Read the model definition and answer for the solid it produces. Units are mm, in the model's axes. A direction names the side the tool comes from. Coordinates: 2 decimals unless noted, no trailing zeros. Write each loop counter-clockwise with the first axis right and the second up, starting at its lowest first coordinate (ties: lowest second). Pieces come first, ordered by that corner, then holes. Notation, with made-up numbers: (52, -13.5) - (91, -13.5) arc R20 ccw to (91, 6.5) - close; hole circle Ø2 at (63, 86). An arc over 180 degrees is marked (long way). Return JSON: item names as keys, results as strings.
```python
from build123d import *

# Parameters (mm, degrees)
EXTRUSION007_DEPTH = 57.9662962441
EXTRUSION006_DEPTH = 1


with BuildPart() as extrusion007:
    # Wire001 → Extrusion007 (new body)
    with BuildSketch(Plane(origin=(-19.0696986475, 108.1739584895, -123.4863420229), x_dir=(1, 0, 0), z_dir=(0, 0, -1))):
        Polygon((0, 0), (18.8765567724, 26.5836913795), (-18.8667640129, 26.5836945158), align=None)
    extrude(amount=-EXTRUSION007_DEPTH)


with BuildPart() as cut:
    # Wire → Extrusion006 (new body)
    with BuildSketch(Plane(origin=(15.2992136515, 73.5902667511, -123.4863420229), x_dir=(1, 0, 0), z_dir=(0, 0, 1))):
        Polygon((0, 0), (-68.7233756416, 0), (-34.3706052198, 48.4038255867), align=None)
    extrude(amount=EXTRUSION006_DEPTH)

    # Cut: cut Extrusion007
    add(extrusion007.part, mode=Mode.SUBTRACT)


solid = cut.part
```
(1) A cutting plane is placed at C-C (y = 92). Determine the outline of the cut face in (x, z), and give its area (3 significant figures).
Answer:
{"outline": "(-40.36, -123.49) - (-30.55, -123.49) - (-30.55, -122.49) - (-40.36, -122.49) - close; (-7.58, -123.49) - (2.23, -123.49) - (2.23, -122.49) - (-7.58, -122.49) - close", "area": "19.6 mm²"}
(2) A cutting plane is placed at A-A (x = -35.5). Determine the outline of the cut face in (y, z), and give its area (3 significant figures).
Answer:
{"outline": "(73.59, -123.49) - (81.59, -123.49) - (81.59, -122.49) - (73.59, -122.49) - close; (85.02, -123.49) - (98.85, -123.49) - (98.85, -122.49) - (85.02, -122.49) - close", "area": "21.8 mm²"}
(3) A cutting plane is placed at D-D (y = 112). Determine the outline of the cut face in (x, z), and give its area (3 significant figures).
Answer:
{"outline": "(-26.16, -123.49) - (-11.97, -123.49) - (-11.97, -122.49) - (-26.16, -122.49) - close", "area": "14.2 mm²"}
(4) Straight lines are drawn through the part: line 1 (Y direction, x = -6, z = -123.15); line 2 (Y direction, x = -6.5, z = -122.95); line 3 (X direction, y = 104, z = -122.9). For each, find the intervals that lie inside material, in ascending order. Write a range as from..to.
Answer:
{"line 1": "73.59..81.59, 89.77..103.59", "line 2": "73.59..81.59, 90.47..104.29", "line 3": "-31.84..-22.03, -16.11..-6.29"}
(5) Determine the mould class of faces 3 (the face through (-21, 80, -122.486)), 4 (the face through (-28.635, 94.696, -122.993)), 5 (the face through (-36.49, 97.45, -122.99)) for opening direction X: +X half, -X half, draft (parallel to the pull), parting line (faces both ways), or undercut.
Answer:
{"face 3": "draft", "face 4": "undercut", "face 5": "-X half"}
(6) A cutting plane is placed at B-B (z = -122.65). Determine the outline of the cut face in (x, y), and give its area (3 significant figures).
Answer:
{"outline": "(-53.42, 73.59) - (15.3, 73.59) - (-19.07, 121.99) - close; hole (-37.94, 81.59) - (-0.19, 81.59) - (-19.07, 108.17) - close", "area": "1,160 mm²"}
(7) Which of the six approach directions +Z, -Z, +X, -X, +Y, -Y give full straight-line access (tool end or side, diameter ignored) to faces 1 (the face through (-21, 80, -123.486)), 2 (the face through (-9.764, 95.068, -122.993))?
Answer:
{"face 1": "-Z, +X, -X, +Y, -Y", "face 2": "+Z, -Z"}
(8) A flat-ended cylindrical pin translates along its axis: P1, Ø0.5, axis at x = -14, z = -123, coming from the +Y side. Find the tip coordinate at first contact, or state that the pin passes through.
Answer:
{"P1": "y = 115.2"}
